```python
from build123d import *

# Parameters (mm, degrees)
BOSS_EXTRUDE1_DEPTH      = 50
BOSS_EXTRUDE1_DEPTH_BACK = 10
SKETCH1_W                = 150
SKETCH1_H                = 160
CUT_EXTRUDE1_DEPTH       = 45
CUT_EXTRUDE1_DEPTH_BACK  = 10
SKETCH3_W                = 134
SKETCH3_H                = 144
SKETCH4_W                = 160
SKETCH4_H                = 140
BOSS_EXTRUDE2_DEPTH      = 55
SKETCH7_W                = 144
SKETCH7_H                = 132
CUT_EXTRUDE3_DEPTH       = 47
SKETCH12_R               = 1.375
CUT_EXTRUDE4_DEPTH       = 6
SKETCH13_R               = 1.375
CUT_EXTRUDE5_DEPTH       = 6
SKETCH16_R               = 1.375
CUT_EXTRUDE6_DEPTH       = 6
SKETCH17_W               = 9
SKETCH17_H               = 11.25
SKETCH17_W_2             = 10.2
SKETCH17_H_2             = 6.2
CUT_EXTRUDE7_DEPTH       = 5
SKETCH18_R               = 3.55
SKETCH18_R_2             = 2.6
SKETCH18_R_3             = 2.35
SKETCH18_W               = 71.34
SKETCH18_H               = 24.5
SKETCH18_W_2             = 21.5
SKETCH18_H_2             = 15.5
CUT_EXTRUDE8_DEPTH       = 15
SKETCH20_W               = 51.644409869
SKETCH20_H               = 15
CUT_EXTRUDE9_DEPTH       = 5
FILLET3_R                = 5
SKETCH21_R               = 2.375
CUT_EXTRUDE10_DEPTH      = 10
SKETCH22_R               = 4.95
SKETCH22_R_2             = 1.375
CUT_EXTRUDE11_DEPTH      = 3
SKETCH23_R               = 1.375
CUT_EXTRUDE12_DEPTH      = 5
SKETCH25_W               = 42.5
SKETCH25_H               = 42.5
CUT_EXTRUDE13_DEPTH      = 60
SKETCH26_W               = 5
SKETCH26_H               = 24
CUT_EXTRUDE14_DEPTH      = 5


with BuildPart() as part:
    # Sketch1 → Boss-Extrude1 (new, two sides: drawn at the far end of the back side and taken through both)
    with BuildSketch(Plane(origin=(0, 0, 0), x_dir=(1, 0, 0), z_dir=(0, 1, 0)).offset(-BOSS_EXTRUDE1_DEPTH_BACK)):
        Rectangle(SKETCH1_W, SKETCH1_H)
    extrude(amount=BOSS_EXTRUDE1_DEPTH + BOSS_EXTRUDE1_DEPTH_BACK)

    # Sketch3 → Cut-Extrude1 (cut, two sides: drawn at the far end of the back side and taken through both)
    with BuildSketch(Plane(origin=(0, 0, 0), x_dir=(1, 0, 0), z_dir=(0, 1, 0)).offset(-CUT_EXTRUDE1_DEPTH_BACK)):
        Rectangle(SKETCH3_W, SKETCH3_H)
    extrude(amount=CUT_EXTRUDE1_DEPTH + CUT_EXTRUDE1_DEPTH_BACK, mode=Mode.SUBTRACT)

    # Sketch4 → Boss-Extrude2 (add)
    with BuildSketch(Plane.ZY.offset(75)):
        with Locations((0, -80)):
            Rectangle(SKETCH4_W, SKETCH4_H)
    extrude(amount=-BOSS_EXTRUDE2_DEPTH)

    # Sketch7 → Cut-Extrude3 (cut)
    with BuildSketch(Plane(origin=(-20, 0, 0), x_dir=(0, 0, -1), z_dir=(1, 0, 0))):
        with Locations((0, -76)):
            Rectangle(SKETCH7_W, SKETCH7_H)
    extrude(amount=-CUT_EXTRUDE3_DEPTH, mode=Mode.SUBTRACT)

    # Sketch12 → Cut-Extrude4 (cut)
    with BuildSketch(Plane(origin=(-20, 0, 0), x_dir=(0, 0, -1), z_dir=(1, 0, 0))):
        with Locations((-76, -146)):
            Circle(SKETCH12_R)
        with Locations((76, -146)):
            Circle(SKETCH12_R)
        with Locations((76, -66)):
            Circle(SKETCH12_R)
        with Locations((-76, -66)):
            Circle(SKETCH12_R)
    extrude(amount=-CUT_EXTRUDE4_DEPTH, mode=Mode.SUBTRACT)

    # Sketch13 → Cut-Extrude5 (cut)
    with BuildSketch(Plane(origin=(0, -10, 0), x_dir=(-1, 0, 0), z_dir=(0, -1, 0))):
        with Locations(Location((-71, 76, 0), (0, 0, 90))):
            Circle(SKETCH13_R)
        with Locations(Location((-6, 76, 0), (0, 0, 90))):
            Circle(SKETCH13_R)
        with Locations(Location((-6, -76, 0), (0, 0, 90))):
            Circle(SKETCH13_R)
        with Locations(Location((-71, -76, 0), (0, 0, 90))):
            Circle(SKETCH13_R)
    extrude(amount=-CUT_EXTRUDE5_DEPTH, mode=Mode.SUBTRACT)

    # Sketch16 → Cut-Extrude6 (cut)
    with BuildSketch(Plane(origin=(0, 45, 0), x_dir=(-1, 0, 0), z_dir=(0, -1, 0))):
        with Locations(Location((18.319208848, -58, 0), (0, 0, 90))):
            Circle(SKETCH16_R)
        with Locations(Location((18.319208848, 24.55, 0), (0, 0, 90))):
            Circle(SKETCH16_R)
        with Locations(Location((-29.940791152, -56.8, 0), (0, 0, 90))):
            Circle(SKETCH16_R)
        with Locations(Location((-29.940791152, 18.13, 0), (0, 0, 90))):
            Circle(SKETCH16_R)
    extrude(amount=-CUT_EXTRUDE6_DEPTH, mode=Mode.SUBTRACT)

    # Sketch17 → Cut-Extrude7 (cut)
    with BuildSketch(Plane.XY.offset(80)):
        with Locations((-11.319208848, 31.775)):
            Rectangle(SKETCH17_W, SKETCH17_H)
        with Locations((12.730791152, 34.3)):
            Rectangle(SKETCH17_W_2, SKETCH17_H_2)
        with Locations((-0.469208848, 34.3)):
            Rectangle(SKETCH17_W_2, SKETCH17_H_2)
    extrude(amount=-CUT_EXTRUDE7_DEPTH, mode=Mode.SUBTRACT)

    # Sketch18 → Cut-Extrude8 (cut)
    with BuildSketch(Plane.ZY.offset(75)):
        with Locations((20, -90.5)):
            Circle(SKETCH18_R)
        with Locations((-19.79104036, -90.5)):
            Circle(SKETCH18_R_2)
        with Locations((0, -15)):
            Circle(SKETCH18_R_3)
        with Locations((0, -117.75)):
            Rectangle(SKETCH18_W, SKETCH18_H)
        with Locations((0, -90.5)):
            Rectangle(SKETCH18_W_2, SKETCH18_H_2)
    extrude(amount=-CUT_EXTRUDE8_DEPTH, mode=Mode.SUBTRACT)

    # Sketch20 → Cut-Extrude9 (cut)
    with BuildSketch(Plane(origin=(0, 0, 72), x_dir=(-1, 0, 0), z_dir=(0, 0, -1))):
        with Locations((-5.002996086, 32.5)):
            Rectangle(SKETCH20_W, SKETCH20_H)
    extrude(amount=-CUT_EXTRUDE9_DEPTH, mode=Mode.SUBTRACT)

    # Fillet3
    # the kernel refuses this fillet: 5 mm, written as the material it adds along each edge
    with BuildSketch(Plane(origin=(-33.319208848, 25, 77), x_dir=(0, 1, 0), z_dir=(1, 0, 0))) as fillet3_piece_1_section:
        with BuildLine():
            CenterArc((FILLET3_R, -FILLET3_R), FILLET3_R, 90, 90)
            Line((0, -FILLET3_R), (0, 0))
            Line((0, 0), (FILLET3_R, 0))
        make_face()
    fillet3_piece_1 = extrude(amount=76.644409869, mode=Mode.PRIVATE)
    fillet3_piece_1 = split(fillet3_piece_1, bisect_by=Plane(origin=(-15.819208848, 27.074193892, 76.479369386), z_dir=(-1, 0, 0)), keep=Keep.TOP, mode=Mode.PRIVATE)
    add(fillet3_piece_1)
    with BuildSketch(Plane(origin=(-33.319208848, 25, 77), x_dir=(0, 1, 0), z_dir=(1, 0, 0))) as fillet3_piece_2_section:
        with BuildLine():
            CenterArc((FILLET3_R, -FILLET3_R), FILLET3_R, 90, 90)
            Line((0, -FILLET3_R), (0, 0))
            Line((0, 0), (FILLET3_R, 0))
        make_face()
    fillet3_piece_2 = extrude(amount=76.644409869, mode=Mode.PRIVATE)
    fillet3_piece_2 = split(fillet3_piece_2, bisect_by=Plane(origin=(-11.319208848, 26.15, 75.492647352), z_dir=(0, -1, 0)), keep=Keep.TOP, mode=Mode.PRIVATE)
    add(fillet3_piece_2)
    with BuildSketch(Plane(origin=(-33.319208848, 25, 77), x_dir=(0, 1, 0), z_dir=(1, 0, 0))) as fillet3_piece_3_section:
        with BuildLine():
            CenterArc((FILLET3_R, -FILLET3_R), FILLET3_R, 90, 90)
            Line((0, -FILLET3_R), (0, 0))
            Line((0, 0), (FILLET3_R, 0))
        make_face()
    fillet3_piece_3 = extrude(amount=76.644409869, mode=Mode.PRIVATE)
    fillet3_piece_3 = split(fillet3_piece_3, bisect_by=Plane(origin=(-6.819208848, 27.074193892, 76.479369386), z_dir=(1, 0, 0)), keep=Keep.TOP, mode=Mode.PRIVATE)
    add(fillet3_piece_3)

    # Sketch21 → Cut-Extrude10 (cut)
    with BuildSketch(Plane(origin=(0, 50, 0), x_dir=(1, 0, 0), z_dir=(0, 1, 0))):
        with Locations(Location((50, 50, 0), (0, 0, 270))):
            Circle(SKETCH21_R)
        with Locations(Location((-30, 50, 0), (0, 0, 270))):
            Circle(SKETCH21_R)
        with Locations(Location((-30, -50, 0), (0, 0, 270))):
            Circle(SKETCH21_R)
        with Locations(Location((50, -50, 0), (0, 0, 270))):
            Circle(SKETCH21_R)
    extrude(amount=-CUT_EXTRUDE10_DEPTH, mode=Mode.SUBTRACT)

    # Sketch22 → Cut-Extrude11 (cut)
    with BuildSketch(Plane.XZ.offset(-45)):
        with Locations(Location((-30, 50, 0), (0, 0, 270))):
            Circle(SKETCH22_R)
        with Locations(Location((50, 50, 0), (0, 0, 270))):
            Circle(SKETCH22_R)
        with Locations(Location((50, -50, 0), (0, 0, 270))):
            Circle(SKETCH22_R)
        with Locations(Location((-30, -50, 0), (0, 0, 270))):
            Circle(SKETCH22_R)
        with Locations(Location((-37, 40, 0), (0, 0, 270))):
            Circle(SKETCH22_R_2)
        with Locations(Location((53, 40, 0), (0, 0, 270))):
            Circle(SKETCH22_R_2)
        with Locations(Location((53, -40, 0), (0, 0, 270))):
            Circle(SKETCH22_R_2)
        with Locations(Location((-37, -40, 0), (0, 0, 270))):
            Circle(SKETCH22_R_2)
    extrude(amount=-CUT_EXTRUDE11_DEPTH, mode=Mode.SUBTRACT)

    # Sketch23 → Cut-Extrude12 (cut)
    with BuildSketch(Plane(origin=(-67, 0, 0), x_dir=(0, 0, -1), z_dir=(1, 0, 0))):
        with Locations((53, -137)):
            Circle(SKETCH23_R)
        with Locations((-53, -137)):
            Circle(SKETCH23_R)
        with Locations((-53, 3)):
            Circle(SKETCH23_R)
        with Locations((53, 3)):
            Circle(SKETCH23_R)
    extrude(amount=-CUT_EXTRUDE12_DEPTH, mode=Mode.SUBTRACT)

    # Sketch25 → Cut-Extrude13 (cut)
    with BuildSketch(Plane.XZ.offset(10)):
        with Locations((69.5, 0)):
            Rectangle(SKETCH25_W, SKETCH25_H)
    extrude(amount=-CUT_EXTRUDE13_DEPTH, mode=Mode.SUBTRACT)

    # Sketch26 → Cut-Extrude14 (cut)
    with BuildSketch(Plane.XZ.offset(-45)):
        with Locations((61.60913212, -33.192475412)):
            Rectangle(SKETCH26_W, SKETCH26_H)
    extrude(amount=-CUT_EXTRUDE14_DEPTH, mode=Mode.SUBTRACT)


solid = part.part
```
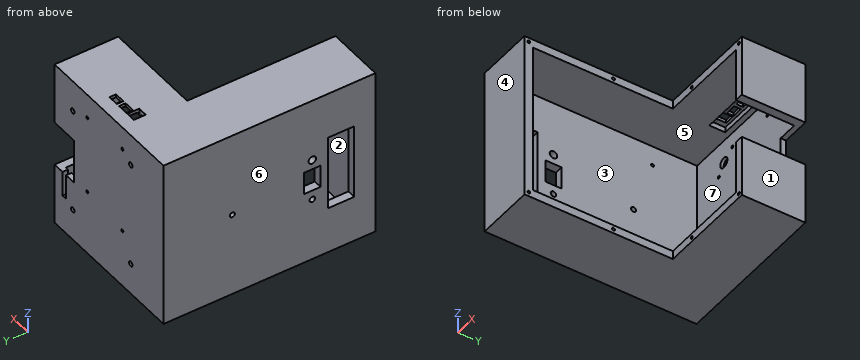
Here's how the part is built. I have some questions about the finished solid (model axes, mm). Face numbers are marked on the shaded views. A direction names the side the tool comes from. Coordinates: 2 decimals unless noted, no trailing zeros. Loops run counter-clockwise (first coordinate to the right, second up) from the corner with the lowest first, then second, coordinate; pieces in that order, holes last. Notation, with made-up numbers: (59.5, 66.25) - (118.5, 66.25) arc R28 cw to (118.5, 96.25) - close; hole circle Ø11 at (-27, 53). An arc over 180 degrees is marked (long way). Answer as CSV lines item,"result".
Q1. If we section it at B-B, the plane z = -8: Write out the boundary of the cut face in (x, y), and give its area (3 significant figures).
Response:
outline,"(-75, -150) - (-20, -150) - (-20, -142) - (-67, -142) - (-67, -130) - (-75, -130) - close; (-75, -105.5) - (-67, -105.5) - (-67, -98.25) - (-75, -98.25) - close; (-75, -82.75) - (-67, -82.75) - (-67, 45) - (48.25, 45) - (48.25, 50) - (-75, 50) - close"
area,"2,230 mm2"
Q2. If we section it at D-D, the plane x = -56: Write out the boundary of the cut face in (y, z), and give its area (3 significant figures).
Response:
outline,"(-150, -80) - (50, -80) - (50, 80) - (-150, 80) - close; hole (-142, -72) - (45, -72) - (45, 72) - (-142, 72) - close"
area,"5,070 mm2"
Q3. We'd pull the mould along Y, two halves only. Please class the marked faces 4, 5, 6 and 7: pulls with the +Y half, pulls with the -Y half, needs draft (parallel to the pull), parting line crosses it, or undercut.
Response:
face 4,"pulls with the -Y half"
face 5,"undercut"
face 6,"needs draft"
face 7,"undercut"
Q4. If we section it at A-A, the plane x = -3: Write out the boundary of the cut face in (y, z), and give its area (3 significant figures).
Response:
outline,"(-10, -80) - (50, -80) - (50, 80) - (37.4, 80) - (37.4, 77) - (40, 77) - (40, 72) - (45, 72) - (45, -72) - (-10, -72) - close; (-10, 72) - (25, 72) arc R5 cw to (30, 77) - (31.2, 77) - (31.2, 80) - (-10, 80) - close"
area,"1,590 mm2"
Q5. For the marked faces 1, 2 and 3, which set-ups out of +Z, -Z, +X, -X, +Y, -Y let a thin tool reach every point of the face, with its end or its side?
Response:
face 1,"+Z, -Z, +X, +Y, -Y"
face 2,"+X"
face 3,"none"
Q6. If we section it at C-C, the plane y = -113: Write out the boundary of the cut face in (x, z).
Response:
outline,"(-75, -80) - (-20, -80) - (-20, -72) - (-67, -72) - (-67, -35.67) - (-75, -35.67) - close; (-75, 35.67) - (-67, 35.67) - (-67, 72) - (-20, 72) - (-20, 80) - (-75, 80) - close"
Q7. For pin 1 (17.5 mm diameter, centred on x = 28.5, z = -63.5, fed in from -Y); pin 2 (3 mm diameter, centred on x = 29.94, z = -18.13, fed in from -Y); pin 3 (0.8 mm diameter, centred on y = -136.5, z = -52.5, fed in from +X), each with a flat end and sliding along its axis, tell me the tip position at first contact or that it passes through.
Response:
pin 1,"y = -10"
pin 2,"y = 45"
pin 3,"x = -72"
Q8. If I drill on L1, parallel to X at y = 47, z = 40 (3 decimals); L2, parallel to X at y = 48.4, z = -50 (3 decimals); L3, parallel to Y at x = -69.8, z = 53 (3 decimals), over which ranges is the centre line in solid material (lowest first)? Write a range as [from, to].
Response:
L1,"[-75, -38.375], [-35.625, 51.625], [54.375, 75]"
L2,"[-75, -32.375], [-27.625, 47.625], [52.375, 75]"
L3,"[-150, -138.375], [-135.625, 1.625], [4.375, 50]"
